Check sheet for the modelled part. Datum: model origin and axes. Units: mm. A direction names the side the tool comes from. Round coordinates to 2 decimals unless told otherwise and drop trailing zeros. Write each loop counter-clockwise with the first axis right and the second up, starting at its lowest first coordinate (ties: lowest second). Pieces come first, ordered by that corner, then holes.
Item 1: Cross-section at D-D on x = 0. Enter the section's corners in (y, z), plus the area to 3 significant figures.
Item 2: Cross-section at B-B on z = 0. Count the separate pieces of the cut face and the enclosed holes in it, plus the area to 3 significant figures.
Item 3: Cross-section at A-A on x = 15.5. Enter the section's corners in (y, z), plus the area to 3 significant figures.
Item 4: Go/stop test with flat-tipped pins: pin 1 Ø2 at (y, z) = (9, 2.5) entering from -X; pin 2 Ø5 at (x, z) = (61.9, 0) entering from +Y; pin 3 Ø6 at (x, z) = (-7.5, 3) entering from +Y; pin 4 Ø5 at (x, z) = (-10, -1.5) entering from -Y. Record where each tip stops, or that it passes through.
Item 5: Material ranges on line 1 (X direction, y = 5, z = -0.5); line 2 (X direction, y = 4.5, z = 2); line 3 (Y direction, x = 37, z = -0.25), recorded low to high.
Item 6: Release check for a two-part mould opening along X. For faces 1 (the flat face through (-71.367, 2, 0)), 2 (the cylindrical face through (-61.744, 1.774, 0.093)), 3 (the flat face through (-21, 0, -2.3)) record: +X half, -X half, draft (parallel to the pull), parting line (faces both ways), or undercut.
Item 7: Tool access check on faces 4 (the flat face through (39, 3.5, 0)), 5 (the cylindrical face through (-0.1, 5.5, -0.1)). Record the directions out of +Z, -Z, +X, -X, +Y, -Y that give a thin tool (end or side, any length) a straight path to the whole face; none if there is none.
Autodesk Fusion 360 part; units mm, degrees
sketch "Sketch1" plane through (0, 0, 0) normal (0, 0, 1) x (1, 0, 0)
  circle A0 centre (-43.925, 0) radius 12.925
  circle A1 centre (-43.925, 0) radius 7.925
  circle A2 centre (0, 0) radius 10.5
  circle A3 centre (0, 0) radius 5.5
  line L0 (9.8995, 3.5) -> (69.8995, 3.5)
  line L1 (69.8995, 3.5) -> (69.8995, -3.5)
  line L2 (69.8995, -3.5) -> (9.8995, -3.5)
  line L3 (-31.5162, 3.6163) -> (-9.7806, 3.8197)
  line L4 (-31.4507, -3.3834) -> (-10.006, -3.1827)
  line L5 (-56.3671, 3.5) -> (-71.3671, 3.5)
  line L6 (-71.3671, 3.5) -> (-71.3671, -3.5)
  line L7 (-71.3671, -3.5) -> (-56.3671, -3.5)
  line L8 (-43.925, 0) -> (0, 0) construction
  dimension "d1" = 3.5
  dimension "d2" = 3.5
  dimension "d3" = 3.5
  dimension "d4" = 3.5
  dimension "d5" = 3.5
  dimension "d6" = 3.5
  dimension "d7" = 43.925
  dimension "d8" = 60
  dimension "d9" = 15
  dimension "d19" = 25.85
  dimension "d20" = 21
  dimension "d21" = 11
  dimension "d22" = 15.85
extrude "Extrude1" add sketch "Sketch1" along normal mid plane 10
sketch "Sketch4" plane through (0, 3.5, 0) normal (0, 1, 0) x (-1, 0, 0)
  line L0 (71.3671, -5) -> (71.3671, 5)
  line L1 (71.3671, 5) -> (56.3671, 5)
  line L2 (56.3671, 5) -> (56.3671, -5)
  line L3 (56.3671, -5) -> (71.3671, -5)
  circle A0 centre (63.8671, 0) radius 2.125
  line L4 (31.5162, -5) -> (9.7806, -5)
  line L5 (31.5162, 5) -> (31.5162, -5)
  line L6 (9.7806, -5) -> (9.7806, 5)
  dimension "d25" = 4.25
  dimension "d27" = 5
  dimension "d31" = 7.5
  dimension "d32" = 7.5
extrude "Extrude4" cut sketch "Sketch4" along normal up to surface contours A0 end surface through (-31.4507, -3.3834, 0) normal (0.009359, -0.999956, 0) offset 0
sketch "Sketch5" plane through (-0.0366, 3.9109, 0) normal (-0.0094, 1, 0) x (0, 0, 1)
  line L0 (-5, -31.481) -> (5, -31.481)
  line L1 (5, -31.481) -> (5, -9.7444)
  line L2 (5, -9.7444) -> (-5, -9.7444)
  line L3 (-5, -9.7444) -> (-5, -31.481)
  circle A0 centre (0, -20.613) radius 2.125
  dimension "d35" = 4.25
  dimension "d36" = 10.868
  dimension "d37" = 10.8686
  dimension "d38" = 5
extrude "Extrude5" cut sketch "Sketch5" against normal up to surface (7 mm away) contours A0
sketch "Sketch6" plane through (0, 3.5, 0) normal (0, 1, 0) x (-1, 0, 0)
  line L0 (-9.8995, -5) -> (-9.8995, 5)
  line L1 (-9.8995, 5) -> (-69.8995, 5)
  line L2 (-69.8995, 5) -> (-69.8995, -5)
  line L3 (-69.8995, -5) -> (-9.8995, -5)
sketch "Sketch7" plane through (0, 3.5, 0) normal (0, 1, 0) x (-1, 0, 0)
  line L0 (-9.8995, -5) -> (-9.8995, 5) construction
  line L1 (-9.8995, 5) -> (-69.8995, 5) construction
  line L2 (-69.8995, 5) -> (-69.8995, -5) construction
  line L3 (-69.8995, -5) -> (-9.8995, -5) construction
  line L4 (-69.8995, 0) -> (-9.8995, 0) construction
  circle A0 centre (-61.8995, 0) radius 2.125
  circle A1 centre (-14.8995, 0) radius 2.125
  dimension "d41" = 4.25
  dimension "d42" = 4.25
  dimension "d43" = 8
  dimension "d44" = 5
extrude "Extrude6" cut sketch "Sketch7" against normal up to surface (7 mm away)
sketch "Sketch3" plane through (0, 0, 0) normal (0, 1, 0) x (1, 0, 0)
  line L0 (-71.3671, 5) -> (-71.3671, -5)
  line L1 (-71.3671, -5) -> (-56.3671, -5)
  line L2 (-56.3671, -5) -> (-56.3671, 5)
  line L3 (-56.3671, 5) -> (-71.3671, 5)
  line L4 (9.8995, 5) -> (9.8995, -5)
  line L5 (9.8995, -5) -> (69.8995, -5)
  line L6 (69.8995, -5) -> (69.8995, 5)
  line L7 (69.8995, 5) -> (9.8995, 5)
  line L8 (-71.3671, 5) -> (69.8995, 5)
  line L9 (69.8995, 5) -> (69.8995, -5)
  line L10 (69.8995, -5) -> (-71.3671, -5)
  line L11 (-71.3671, -5) -> (-71.3671, 5)
  circle A0 centre (-63.8671, 0) radius 2.125
  circle A1 centre (14.8995, 0) radius 2.125
  circle A2 centre (61.8995, 0) radius 2.125
extrude "Extrude3" cut sketch "Sketch3" against normal blind 20 contours L0 L1 L2 L3 L8 L10 L11 | L2 L4 L8 L10 | L4 L5 L6 L7 L8 L9 L10 | A0 | A1 | A2
equation "d2 = d1"
equation "d3 = d1"
equation "d4 = d1"
equation "d5 = d1"
equation "d6 = d1"
equation "d42 = d41"
Response values:
1. outline: (5.5, -5) - (10.5, -5) - (10.5, 5) - (5.5, 5) - close
1. area: 50.0 mm2
2. separate pieces: 4
2. enclosed holes: 0
2. area: 567 mm2
3. outline: (0, -5) - (3.5, -5) - (3.5, -2.04) - (0, -2.04) - close; (0, 2.04) - (3.5, 2.04) - (3.5, 5) - (0, 5) - close
3. area: 20.7 mm2
4. pin 1: stops at x = -54.08
4. pin 2: stops at y = 3.5
4. pin 3: stops at y = 9.49
4. pin 4: stops at y = 0
5. line 1: x = -55.84 to -50.07, -37.78 to -32.01, -9.23 to -2.29, 2.29 to 9.23
5. line 2: x = -56.04 to -50.45, -37.4 to -31.81, -9.49 to -3.16, 3.16 to 9.49
5. line 3: y = 0 to 3.5
6. face 1: -X half
6. face 2: undercut
6. face 3: draft
7. face 4: +Z, -Z, +X, +Y
7. face 5: +Z, -Z, -Y
